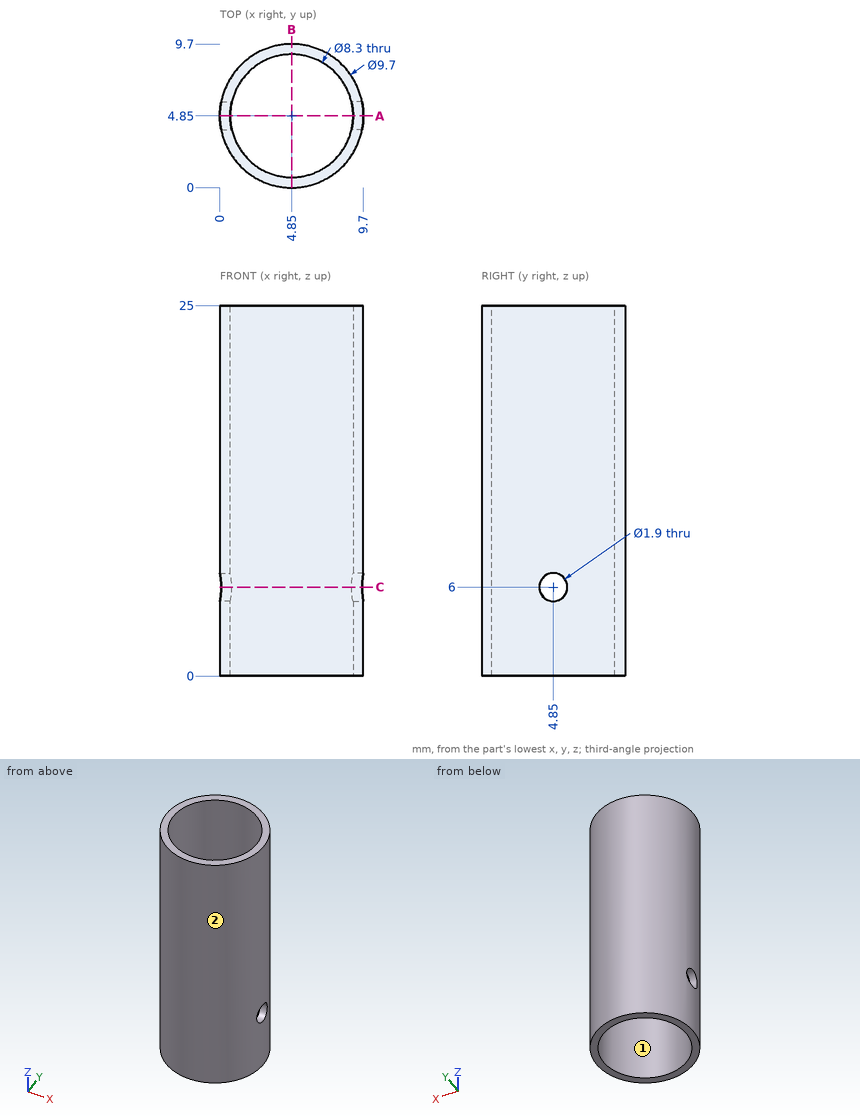
Can you work these out from the drawing? Everything is in mm from the part's minimum corner. Round coordinates to 2 decimals unless told otherwise and drop trailing zeros. Order: outer loops, then holes, each group sorted by start corner. A loop starts at its lowest first (then second) coordinate and runs counter-clockwise, first axis right, second up. Notation, with made-up numbers: (-24.5, -29.75) -> (22.5, -29.75) arc R27 ccw to (22.5, -13.75) -> close; hole circle Ø2 at (-11.75, 65). An arc over 180 degrees is marked (long way). Return JSON: item names as keys, results as strings. Group by question number.
1. If we section it at C-C, the plane z = 6: Write out the boundary of the cut face in (x, y), then the cut area to 3 significant figures.
2. Will these pins go through, and if not, where does the flat tip stop? pin 1 (1 mm diameter, centred on x = 2.5, y = 7, fed in from +Z); pin 2 (1 mm diameter, centred on x = 6, z = 19, fed in from +Y); pin 3 (1.5 mm diameter, centred on y = 8, z = 22, fed in from -X); pin 4 (3 mm diameter, centred on y = 2.5, z = 13, fed in from +X).
3. If we section it at A-A, the plane y = 4.85: Write out the boundary of the cut face in (x, z).
4. We'd pull the mould along X, two halves only. Please class the marked faces 1 and 2: released by +X, released by -X, zero draft, split by the parting line, or undercut.
5. If we section it at B-B, the plane x = 4.85: Write out the boundary of the cut face in (y, z).
6. I need wall thicknesses on line 1 (X direction, y = 5, z = 1.5); line 2 (X direction, y = 7.5, z = 17.25). Which ranges of each line are inside material? Lowest first, please. Write a range as [from, to].
Output values:
{
 "1": {"outline": "(0.09, 3.9) arc R4.85 ccw to (9.61, 3.9) -> (8.89, 3.9) arc R4.15 cw to (0.81, 3.9) -> close; (0.09, 5.8) -> (0.81, 5.8) arc R4.15 cw to (8.89, 5.8) -> (9.61, 5.8) arc R4.85 ccw to start", "area": "17.1 mm²"},
 "2": {"pin 1": "through", "pin 2": "y = 9.66", "pin 3": "x = 0.64", "pin 4": "x = 9.62"},
 "3": {"outline": "(0, 0) -> (0.7, 0) -> (0.7, 5.05) -> (0, 5.05) -> close; (0, 6.95) -> (0.7, 6.95) -> (0.7, 25) -> (0, 25) -> close; (9, 0) -> (9.7, 0) -> (9.7, 5.05) -> (9, 5.05) -> close; (9, 6.95) -> (9.7, 6.95) -> (9.7, 25) -> (9, 25) -> close"},
 "4": {"face 1": "undercut", "face 2": "split by the parting line"},
 "5": {"outline": "(0, 0) -> (0.7, 0) -> (0.7, 25) -> (0, 25) -> close; (9, 0) -> (9.7, 0) -> (9.7, 25) -> (9, 25) -> close"},
 "6": {"line 1": "[0, 0.7], [9, 9.7]", "line 2": "[0.79, 1.66], [8.04, 8.91]"}
}
